Geometry check sheet. Reference: drawing and pictorial views, mm from the part's lowest x, y, z. Coordinates: 2 decimals unless noted, no trailing zeros. Loops run counter-clockwise (first coordinate to the right, second up) from the corner with the lowest first, then second, coordinate; pieces in that order, holes last. Notation, with made-up numbers: (43, 31) -> (69, 31) arc R18 ccw to (69, 37) -> close; hole circle Ø1 at (31.25, -21.5). An arc over 180 degrees is marked (long way). Answer as a JSON object with one key per item and string values.
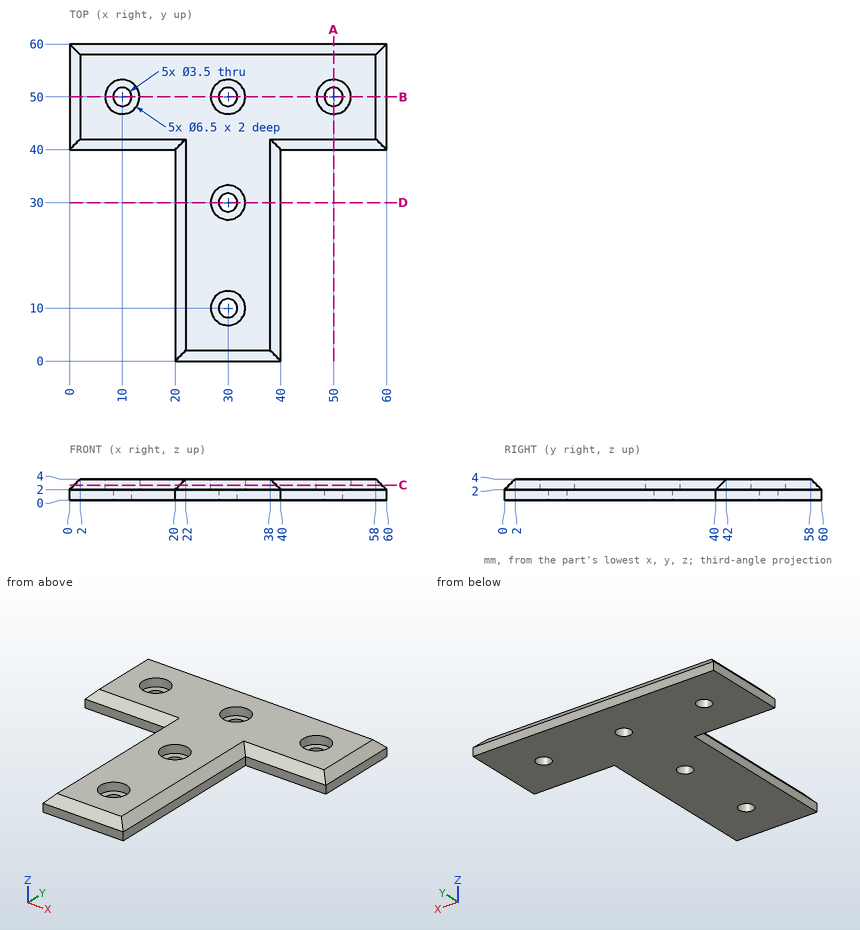
1. Thickness scan on probe 1 along Y at (x, z) = (30, 0.6); probe 2 along Y at (x, z) = (10, 0.65); probe 3 along Y at (x, z) = (30, 3.15). Record the ranges inside material, lowest first. Write a range as from..to.
Evaluation:
{"probe 1": "y = 0..8.25, 11.75..28.25, 31.75..48.25, 51.75..60", "probe 2": "y = 40..48.25, 51.75..60", "probe 3": "y = 1.15..6.75, 13.25..26.75, 33.25..46.75, 53.25..58.85"}
2. Section check A-A, the plane x = 50. Record the boundary of the cut face in (y, z).
Evaluation:
{"outline": "(40, 0) -> (48.25, 0) -> (48.25, 2) -> (46.75, 2) -> (46.75, 4) -> (42, 4) -> (40, 2) -> close; (51.75, 0) -> (60, 0) -> (60, 2) -> (58, 4) -> (53.25, 4) -> (53.25, 2) -> (51.75, 2) -> close"}
3. Section check D-D, the plane y = 30. Record the boundary of the cut face in (x, z), then the cut area to 3 significant figures.
Evaluation:
{"outline": "(20, 0) -> (28.25, 0) -> (28.25, 2) -> (26.75, 2) -> (26.75, 4) -> (22, 4) -> (20, 2) -> close; (31.75, 0) -> (40, 0) -> (40, 2) -> (38, 4) -> (33.25, 4) -> (33.25, 2) -> (31.75, 2) -> close", "area": "56.0 mm^2"}
4. Section check C-C, the plane z = 2.85. Record the boundary of the cut face in (x, y), then the cut area to 3 significant figures.
Evaluation:
{"outline": "(0.85, 40.85) -> (20.85, 40.85) -> (20.85, 0.85) -> (39.15, 0.85) -> (39.15, 40.85) -> (59.15, 40.85) -> (59.15, 59.15) -> (0.85, 59.15) -> close; hole circle Ø6.5 at (10, 50); hole circle Ø6.5 at (30, 10); hole circle Ø6.5 at (30, 30); hole circle Ø6.5 at (30, 50); hole circle Ø6.5 at (50, 50)", "area": "1,630 mm^2"}
5. Section check B-B, the plane y = 50. State how many separate pieces and enclosed holes the cut face has, then the cut area to 3 significant figures.
Evaluation:
{"separate pieces": "4", "enclosed holes": "0", "area": "176 mm^2"}
6. Depth check by flat-ended pin: P1, Ø1.5, axis at x = 17.5, z = 1.5, coming from the -Y side; P2, Ø4, axis at x = 30, y = 10, coming from the +Z side; P3, Ø1.6, axis at y = 10, z = 1.5, coming from the +X side; P4, Ø2, axis at x = 30.5, y = 10.5, coming from the -Z side. Enter the tip coordinate at first touch or a pass-through.
Evaluation:
{"P1": "stops at y = 40", "P2": "stops at z = 2", "P3": "stops at x = 40", "P4": "passes through"}
